Drawing for the job (mm, zero at the part's lowest x, y, z). A direction names the side the tool comes from. Give positions to 0.01 mm unless a question says otherwise; leave off trailing zeros. Write each loop counter-clockwise with the first axis right and the second up, starting at its lowest first coordinate (ties: lowest second). Pieces come first, ordered by that corner, then holes. Notation, with made-up numbers: M -34.5,52 L 10.5,52 A28 cw 10.5,80 Z; hole C 6,-19 d11. An arc over 180 degrees is marked long. Write item = value, one per line. Start each with the question number.
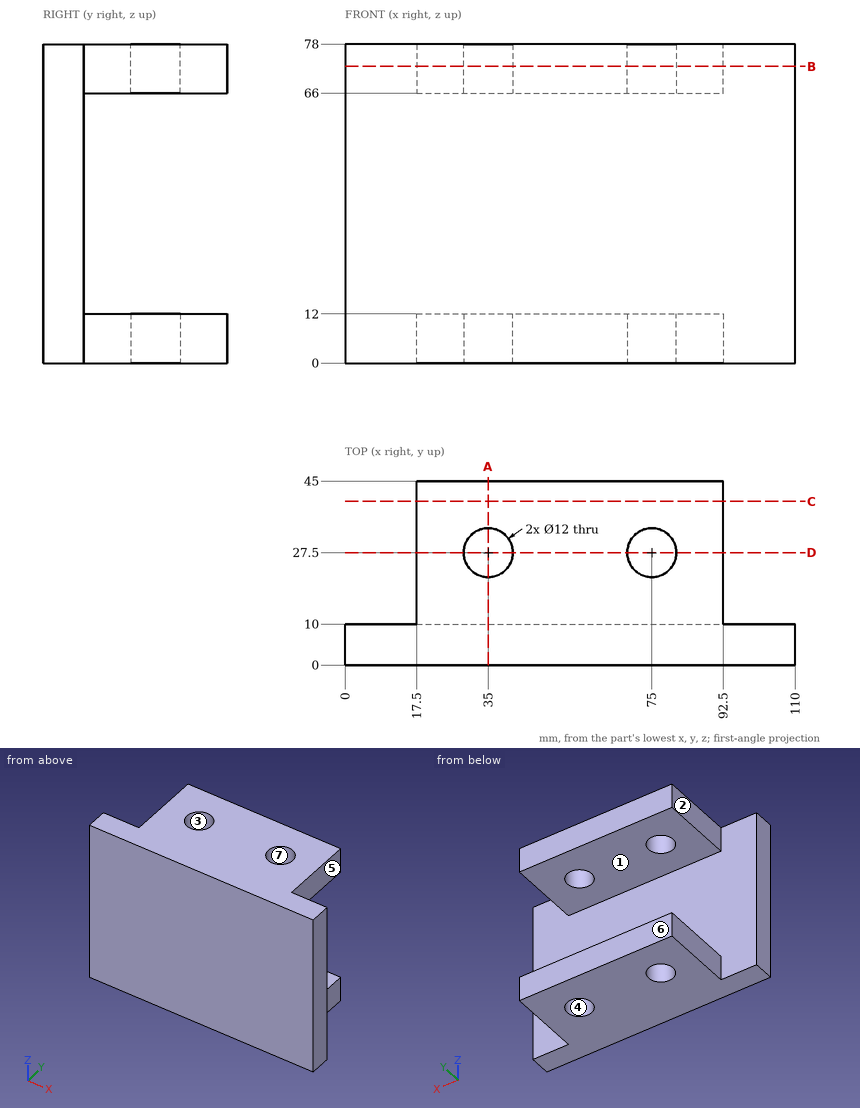
Q1. Slice it at D-D (y = 27.5). Give the cut face in (x, z).
Q2. Probe line 1 along X through (y, z) = (27, 3); line 2 along Z through (x, y) = (50.5, 20); line 3 along Y through (x, z) = (75, 75). List the from-to ranges inside material, lowest first.
Q3. Slice it at A-A (x = 35). Give the cut face in (y, z), and give its area (3 significant figures).
Q4. Slice it at B-B (z = 72.5). Give the cut face in (x, y).
Q5. Drop flat-ended pins along their axis: P1, Ø10, axis at y = 17.5, z = 35, coming from the -X side; P2, Ø15.5, axis at x = 75, y = 27.5, coming from the -Z side; P3, Ø3.5, axis at y = 27.5, z = 71, coming from the +X side; P4, Ø1.5, axis at x = 53, z = 40, coming from the +Y side. Give the stop position or say it passes through.
Q6. Slice it at C-C (y = 40). Give the cut face in (x, z).
Q7. Two-plate mould, pull along X, no slides. Class the marked faces 4, 5, 6 and 7: +X half, -X half, draft (parallel to the pull), parting line (faces both ways), or undercut.
Q8. Tool access for the marked faces 1, 2 and 3: list every direction of +Z, -Z, +X, -X, +Y, -Y with a clear straight run to the whole face (end or side of a thin tool).
Working result:
q1.outline = M 17.5,0 L 29,0 L 29,12 L 17.5,12 Z; M 17.5,66 L 29,66 L 29,78 L 17.5,78 Z; M 41,0 L 69,0 L 69,12 L 41,12 Z; M 41,66 L 69,66 L 69,78 L 41,78 Z; M 81,0 L 92.5,0 L 92.5,12 L 81,12 Z; M 81,66 L 92.5,66 L 92.5,78 L 81,78 Z
q2.line_1 = 17.5 to 29.02, 40.98 to 69.02, 80.98 to 92.5
q2.line_2 = 0 to 12, 66 to 78
q2.line_3 = 0 to 21.5, 33.5 to 45
q3.outline = M 0,0 L 21.5,0 L 21.5,12 L 10,12 L 10,66 L 21.5,66 L 21.5,78 L 0,78 Z; M 33.5,0 L 45,0 L 45,12 L 33.5,12 Z; M 33.5,66 L 45,66 L 45,78 L 33.5,78 Z
q3.area = 1,330 mm2
q4.outline = M 0,0 L 110,0 L 110,10 L 92.5,10 L 92.5,45 L 17.5,45 L 17.5,10 L 0,10 Z; hole C 35,27.5 d12; hole C 75,27.5 d12
q5.P1 = through
q5.P2 = 0
q5.P3 = 92.5
q5.P4 = 10
q6.outline = M 17.5,0 L 92.5,0 L 92.5,12 L 17.5,12 Z; M 17.5,66 L 92.5,66 L 92.5,78 L 17.5,78 Z
q7.face_4 = undercut
q7.face_5 = +X half
q7.face_6 = draft
q7.face_7 = undercut
q8.face_1 = +X, -X, +Y
q8.face_2 = +Z, -Z, -X, +Y
q8.face_3 = +Z, -Z
